Work out the finished part from the listing and answer in its coordinate system (mm). Face numbers are marked on the shaded views. Round coordinates to 2 decimals unless told otherwise and drop trailing zeros. Loops run counter-clockwise (first coordinate to the right, second up) from the corner with the lowest first, then second, coordinate; pieces in that order, holes last.
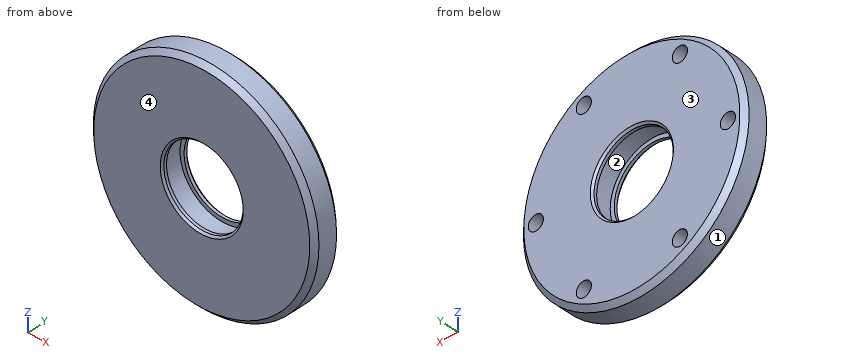
from build123d import *

# Parameters (mm, degrees)
SKETCH1_R           = 23.5
SKETCH1_R_2         = 1.575
SKETCH1_R_3         = 8.25
BOSS_EXTRUDE1_DEPTH = 3
SKETCH2_R           = 9.1
CUT_EXTRUDE1_DEPTH  = 2
SKETCH3_R           = 21.575
SKETCH3_R_2         = 18.425
BOSS_EXTRUDE2_DEPTH = 1
CHAMFER1_SIZE       = 1
CHAMFER2_SIZE       = 0.4


with BuildPart() as part:
    # Sketch1 → Boss-Extrude1 (new body, symmetric)
    with BuildSketch(Plane(origin=(0, 0, 0), x_dir=(1, 0, 0), z_dir=(0, 1, 0))):
        Circle(SKETCH1_R)
        with Locations((20, 0)):
            Circle(SKETCH1_R_2, mode=Mode.SUBTRACT)
        with Locations((10, -17.320508076)):
            Circle(SKETCH1_R_2, mode=Mode.SUBTRACT)
        with Locations((-10, -17.320508076)):
            Circle(SKETCH1_R_2, mode=Mode.SUBTRACT)
        with Locations((-20, 0)):
            Circle(SKETCH1_R_2, mode=Mode.SUBTRACT)
        with Locations((-10, 17.320508076)):
            Circle(SKETCH1_R_2, mode=Mode.SUBTRACT)
        with Locations((10, 17.320508076)):
            Circle(SKETCH1_R_2, mode=Mode.SUBTRACT)
        Circle(SKETCH1_R_3, mode=Mode.SUBTRACT)
    extrude(amount=BOSS_EXTRUDE1_DEPTH, both=True)

    # Sketch2 → Cut-Extrude1 (cut, symmetric)
    with BuildSketch(Plane(origin=(0, 0, 0), x_dir=(1, 0, 0), z_dir=(0, 1, 0))):
        Circle(SKETCH2_R)
    extrude(amount=CUT_EXTRUDE1_DEPTH, both=True, mode=Mode.SUBTRACT)

    # Sketch3 → Boss-Extrude2 (add)
    with BuildSketch(Plane(origin=(0, -3, 0), x_dir=(1, 0, 0), z_dir=(0, 1, 0))):
        Circle(SKETCH3_R)
        Circle(SKETCH3_R_2, mode=Mode.SUBTRACT)
    extrude(amount=BOSS_EXTRUDE2_DEPTH)

    # Chamfer1
    chamfer1_edges = [part.edges().sort_by_distance(p)[0] for p in [
        (-23.5, -3, 0),
        (-23.5, 3, 0),
    ]]
    chamfer(chamfer1_edges, length=CHAMFER1_SIZE)

    # Chamfer2
    chamfer2_edges = [part.edges().sort_by_distance(p)[0] for p in [
        (-8.25, -3, 0),
        (-8.25, 3, 0),
    ]]
    chamfer(chamfer2_edges, length=CHAMFER2_SIZE)


solid = part.part
Item 1: Determine the mould class of the marked faces 1, 2, 3 and 4 for opening direction Y: pulls with the +Y half, pulls with the -Y half, needs draft (parallel to the pull), parting line crosses it, or undercut.
Item 2: Section A-A, the plane x = 0 is taken. Give the vertices of the cut face in (y, z), plus the area to 3 significant figures.
Item 3: Each of these flat-tipped pins is pushed along its axis until it touches: P1, Ø1.6, axis at x = 10, z = 17.5, coming from the +Y side; P2, Ø3.5, axis at x = -19.5, z = 0, coming from the +Y side; P3, Ø1.5, axis at x = 9, y = 0.5, coming from the +Z side; P4, Ø1, axis at x = 2, y = -1.5, coming from the -Z side. Where does it stop, or does it pass through?
Item 4: Straight lines are drawn through the part: line 1 (X direction, y = 1.3, z = 0) (3 decimals); line 2 (Z direction, x = 10, y = 0.45); line 3 (Y direction, x = -3.5, z = 8). For each, find the intervals that lie inside material, in ascending order.
Item 5: Section B-B, the plane y = -1.2 is taken. State how many separate pieces and enclosed holes the cut face has, plus the area to 3 significant figures.
Answer below:
1. face 1: needs draft
1. face 2: undercut
1. face 3: pulls with the +Y half
1. face 4: pulls with the -Y half
2. outline: (-3, -22.5) - (-2, -23.5) - (2, -23.5) - (3, -22.5) - (3, -8.65) - (2.6, -8.25) - (2, -8.25) - (2, -9.1) - (-2, -9.1) - (-2, -8.25) - (-2.6, -8.25) - (-3, -8.65) - close; (-3, 8.65) - (-2.6, 8.25) - (-2, 8.25) - (-2, 9.1) - (2, 9.1) - (2, 8.25) - (2.6, 8.25) - (3, 8.65) - (3, 22.5) - (2, 23.5) - (-2, 23.5) - (-3, 22.5) - close
2. area: 174 mm2
3. P1: stops at y = -2
3. P2: stops at y = 3
3. P3: stops at z = 22
3. P4: stops at z = -23.45
4. line 1: x = -23.5 to -21.575, -18.425 to -9.1, 9.1 to 18.425, 21.575 to 23.5
4. line 2: z = -21.27 to -18.9, -15.75 to 15.75, 18.9 to 21.27
4. line 3: y = -3 to -2, 2 to 3
5. separate pieces: 1
5. enclosed holes: 7
5. area: 1,430 mm2
